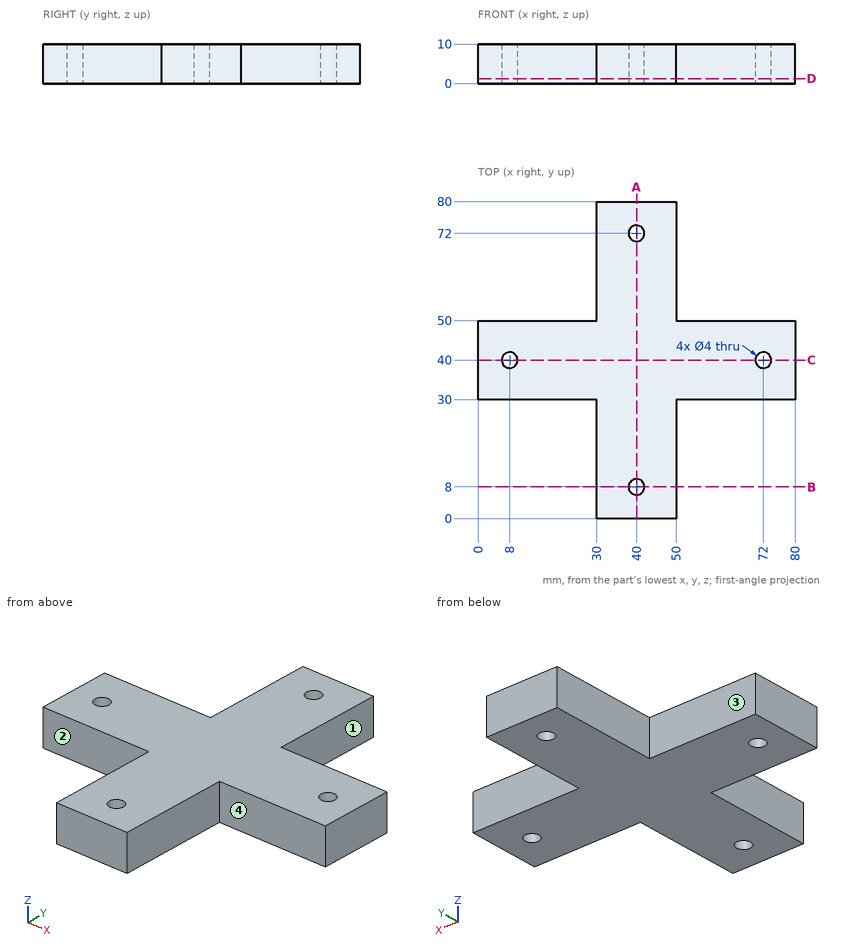
Source: three-view drawing plus pictorial views. Frame: mm from the lowest corner of the part. A direction names the side the tool comes from. Give positions to 0.01 mm unless a question says otherwise; leave off trailing zeros. Order: outer loops, then holes, each group sorted by start corner. A loop starts at its lowest first (then second) coordinate and runs counter-clockwise, first axis right, second up. Notation, with made-up numbers: (63.25, 44.25) -> (82.25, 44.25) arc R29 cw to (82.25, 70.25) -> close; hole circle Ø1 at (-36, -20). An arc over 180 degrees is marked (long way). Write each question's results on one line, items separated by ' | '. Start each with the question number.
Item 1: Cut plane D-D on z = 1.25. Return the cut outline in (x, y).
Item 2: Set-up query: the marked faces 1, 2, 3 and 4. Return all of +Z, -Z, +X, -X, +Y, -Y with unobstructed straight access to the full face (end or side cutting, diameter ignored); none if empty.
Item 3: Cut plane A-A on x = 40. Return the cut outline in (y, z), then the cut area to 3 significant figures.
Item 4: Line query: line 1 (Y direction, x = 40, z = 4); line 2 (X direction, y = 72, z = 7.25); line 3 (X direction, y = 11.5, z = 9.25). Output: solid intervals per line, ascending.
Item 5: Cut plane B-B on y = 8. Return the cut outline in (x, z).
Item 6: Contact query for flat-ended pins moving along their axis: P1, Ø3, axis at x = 40, y = 8, coming from the -Z side; P2, Ø2, axis at x = 16.5, z = 7, coming from the -Y side; P3, Ø5, axis at x = 72, y = 40, coming from the -Z side; P4, Ø5, axis at y = 64.5, z = 5.5, coming from the +X side. Output: stop coordinate, or through.
Established:
1) outline: (0, 30) -> (30, 30) -> (30, 0) -> (50, 0) -> (50, 30) -> (80, 30) -> (80, 50) -> (50, 50) -> (50, 80) -> (30, 80) -> (30, 50) -> (0, 50) -> close; hole circle Ø4 at (8, 40); hole circle Ø4 at (40, 8); hole circle Ø4 at (40, 72); hole circle Ø4 at (72, 40)
2) face 1: +Z, -Z, +X, +Y | face 2: +Z, -Z, -X, -Y | face 3: +Z, -Z, -X, +Y | face 4: +Z, -Z, +X, -Y
3) outline: (0, 0) -> (6, 0) -> (6, 10) -> (0, 10) -> close; (10, 0) -> (70, 0) -> (70, 10) -> (10, 10) -> close; (74, 0) -> (80, 0) -> (80, 10) -> (74, 10) -> close | area: 720 mm^2
4) line 1: 0 to 6, 10 to 70, 74 to 80 | line 2: 30 to 38, 42 to 50 | line 3: 30 to 50
5) outline: (30, 0) -> (38, 0) -> (38, 10) -> (30, 10) -> close; (42, 0) -> (50, 0) -> (50, 10) -> (42, 10) -> close
6) P1: through | P2: y = 30 | P3: z = 0 | P4: x = 50
